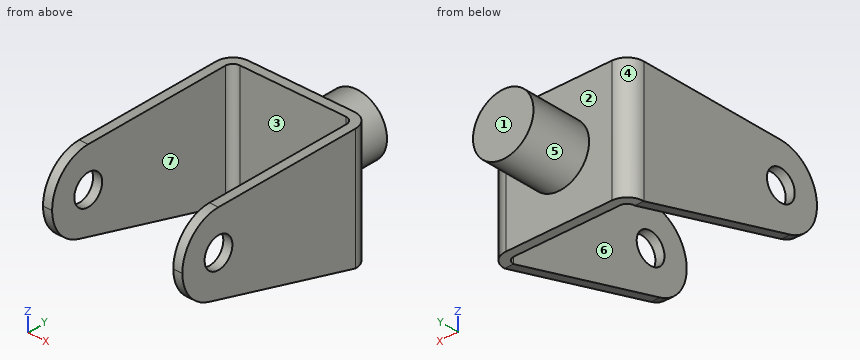
```python
from build123d import *

# Parameters (mm, degrees)
BASE_FLANGE1_DEPTH  = 50.8
SKETCH8_R           = 12.7
CUT_EXTRUDE2_DEPTH  = 215.217642934
SKETCH9_R           = 25.36182522
BOSS_EXTRUDE1_DEPTH = 50.8


# Sheet-metal steps are written as plain solids
with BuildPart() as part:
    # Sketch2 → Base-Flange1 (new, symmetric)
    with BuildSketch(Plane.XY):
        with BuildLine():
            Line((50.8, 0), (50.8, 158.242))
            ThreePointArc((50.8, 158.242), (48.940128061, 162.732128061), (44.45, 164.592))
            Line((44.45, 164.592), (-44.45, 164.592))
            ThreePointArc((-44.45, 164.592), (-48.940128061, 162.732128061), (-50.8, 158.242))
            Line((-50.8, 158.242), (-50.8, 0))
            Line((-50.8, 0), (-58.42, 0))
            Line((-58.42, 0), (-58.42, 158.242))
            ThreePointArc((-58.42, 158.242), (-54.328281733, 168.120281733), (-44.45, 172.212))
            Line((-44.45, 172.212), (44.45, 172.212))
            ThreePointArc((44.45, 172.212), (54.328281733, 168.120281733), (58.42, 158.242))
            Line((58.42, 158.242), (58.42, 0))
            Line((58.42, 0), (50.8, 0))
        make_face()
    extrude(amount=BASE_FLANGE1_DEPTH, both=True)

    # Sketch8 → Cut-Extrude2 (cut, through all)
    with BuildSketch(Plane(origin=(58.42, 0, 0), x_dir=(0, 0, -1), z_dir=(1, 0, 0))):
        with BuildLine():
            Line((50.8, 0), (50.8, 158.242))
            Line((50.8, 158.242), (14.064244739, 24.287046492))
            ThreePointArc((14.064244739, 24.287046492), (2.244463478, 6.764690776), (-17.78, 0))
            Line((-17.78, 0), (50.8, 0))
        make_face()
        with BuildLine():
            Line((-50.8, 0), (-17.78, 0))
            ThreePointArc((-17.78, 0), (-41.128665915, 9.671334085), (-50.8, 33.02))
            Line((-50.8, 33.02), (-50.8, 0))
        make_face()
        with Locations((-17.78, 33.02)):
            Circle(SKETCH8_R)
    extrude(amount=-CUT_EXTRUDE2_DEPTH, mode=Mode.SUBTRACT)

    # Sketch9 → Boss-Extrude1 (add)
    with BuildSketch(Plane(origin=(0, 172.212, 0), x_dir=(1, 0, 0), z_dir=(0, 1, 0))):
        with Locations(Location((0, 0, 0), (0, 0, 270))):
            Circle(SKETCH9_R)
    extrude(amount=BOSS_EXTRUDE1_DEPTH)


solid = part.part
```
Could you check a few things on this model? Use its own coordinates, in mm. Face numbers are marked on the shaded views. A direction names the side the tool comes from. Round coordinates to 2 decimals unless told otherwise and drop trailing zeros. Write each loop counter-clockwise with the first axis right and the second up, starting at its lowest first coordinate (ties: lowest second). Pieces come first, ordered by that corner, then holes. Notation, with made-up numbers: M 72.25,68 L 105.25,68 A15 cw 105.25,74 Z; hole C -5,13 d11. An arc over 180 degrees is marked long. Answer in a Markdown table with one row per item. Add a question column.
Q1. Imagine slicing it at D-D (y = 61.5). Please give me the cut outline in (x, z).
Q2. If we mould it in two halves opening along X, with no side actions, what happens to the marked faces 4, 5, 6 and 7? For each: +X half, -X half, draft (parallel to the pull), parting line (faces both ways), or undercut.
Q3. If I drill on line 1 (X direction, y = 77.5, z = 43.5); line 2 (Y direction, x = 44.5, z = 9); line 3 (Z direction, x = 1, y = 177), over which ranges is the centre line in solid material (lowest first)? Write a range as from..to.
Q4. On a 3-axis mill with a long thin cutter (end or side, diameter ignored), from which of +Z, -Z, +X, -X, +Y, -Y can I reach the whole of each face in a straight line? I mean the marked faces 1, 2 and 3. Say none if no direction works.
Q5. Imagine slicing it at A-A (y = 134.5). Please give me the cut outline in (x, z).
Q6. Imagine slicing it at C-C (z = 0). Please give me the cut outline in (x, y), then the cut area to 3 significant figures.
Q7. Will these pins go through, and if not, where does the flat tip stop? pin 1 Ø4 at (y, z) = (186, 21.5) entering from +X; pin 2 Ø10 at (x, z) = (-3.5, 15) entering from -Y; pin 3 Ø6 at (x, z) = (-41, 8.5) entering from +Y.
Q8. Imagine slicing it at B-B (x = 0). Please give me the cut outline in (y, z).
Values:
| question | item | result |
|---|---|---|
| 1 | outline | M -58.42,-24.27 L -50.8,-24.27 L -50.8,50.8 L -58.42,50.8 Z; M 50.8,-24.27 L 58.42,-24.27 L 58.42,50.8 L 50.8,50.8 Z |
| 2 | face 4 | -X half |
| 2 | face 5 | parting line |
| 2 | face 6 | undercut |
| 2 | face 7 | undercut |
| 3 | line 1 | -58.42..-50.8, 50.8..58.42 |
| 3 | line 2 | 164.59..172.21 |
| 3 | line 3 | -25.34..25.34 |
| 4 | face 1 | +Z, -Z, +X, -X, +Y |
| 4 | face 2 | +Y |
| 4 | face 3 | +Z, -Z, -Y |
| 5 | outline | M -58.42,-44.29 L -50.8,-44.29 L -50.8,50.8 L -58.42,50.8 Z; M 50.8,-44.29 L 58.42,-44.29 L 58.42,50.8 L 50.8,50.8 Z |
| 6 | outline | M -58.42,5.2 L -50.8,5.2 L -50.8,158.24 A6.35 cw -44.45,164.59 L 44.45,164.59 A6.35 cw 50.8,158.24 L 50.8,5.2 L 58.42,5.2 L 58.42,158.24 A13.97 ccw 44.45,172.21 L 25.36,172.21 L 25.36,223.01 L -25.36,223.01 L -25.36,172.21 L -44.45,172.21 A13.97 ccw -58.42,158.24 Z |
| 6 | area | 5,830 mm^2 |
| 7 | pin 1 | x = 16.22 |
| 7 | pin 2 | y = 164.59 |
| 7 | pin 3 | y = 172.21 |
| 8 | outline | M 164.59,-50.8 L 172.21,-50.8 L 172.21,-25.36 L 223.01,-25.36 L 223.01,25.36 L 172.21,25.36 L 172.21,50.8 L 164.59,50.8 Z |
